Autodesk Inventor part; units mm, degrees
ref_plane "to_rail_XY" through (0.6, 10, 200) normal (0, 0, 1) x (1, 0, 0)
ref_plane "to_rail_YZ" through (0.6, 10, 200) normal (1, 0, 0) x (0, 1, 0)
ref_plane "to_rail_ZX" through (0.6, 10, 200) normal (0, 1, 0) x (0, 0, 1)
sketch "Sketch_1" plane through (0, 0, 0) normal (0, 0, 1) x (1, 0, 0)
  line L0 (-7.4, 19.7) -> (-7.4, 0.3)
  arc A0 (-7.4, 0.3) -> (-7.1, 0) centre (-7.1, 0.3) ccw
  line L1 (-7.1, 0) -> (-0.3, 0)
  arc A1 (-0.3, 0) -> (0, 0.3) centre (-0.3, 0.3) ccw
  line L2 (0, 0.3) -> (0, 2.95)
  arc A2 (0, 2.95) -> (-0.2, 3.15) centre (-0.2, 2.95) ccw
  line L3 (-0.2, 3.15) -> (-0.5141, 3.15)
  arc A3 (-0.5141, 3.15) -> (-0.708, 2.999) centre (-0.5141, 2.95) ccw
  arc A4 (-4.392, 2.999) -> (-0.708, 2.999) centre (-2.55, 3.465) ccw
  arc A5 (-4.392, 2.999) -> (-4.5859, 3.15) centre (-4.5859, 2.95) ccw
  line L4 (-4.5859, 3.15) -> (-5.8, 3.15)
  arc A6 (-6, 3.35) -> (-5.8, 3.15) centre (-5.8, 3.35) ccw
  line L5 (-6, 3.35) -> (-6, 16.65)
  arc A7 (-5.8, 16.85) -> (-6, 16.65) centre (-5.8, 16.65) ccw
  line L6 (-5.8, 16.85) -> (-4.5859, 16.85)
  arc A8 (-4.5859, 16.85) -> (-4.392, 17.001) centre (-4.5859, 17.05) ccw
  arc A9 (-0.708, 17.001) -> (-4.392, 17.001) centre (-2.55, 16.535) ccw
  arc A10 (-0.708, 17.001) -> (-0.5141, 16.85) centre (-0.5141, 17.05) ccw
  line L7 (-0.5141, 16.85) -> (-0.2, 16.85)
  arc A11 (-0.2, 16.85) -> (0, 17.05) centre (-0.2, 17.05) ccw
  line L8 (0, 17.05) -> (0, 19.7)
  arc A12 (0, 19.7) -> (-0.3, 20) centre (-0.3, 19.7) ccw
  line L9 (-0.3, 20) -> (-7.1, 20)
  arc A13 (-7.1, 20) -> (-7.4, 19.7) centre (-7.1, 19.7) ccw
extrude "Extrusion1" add sketch "Sketch_1" along normal blind 400
sketch "Sketch2" plane through (-6, 3.35, 0) normal (1, 0, 0) x (0, 0, -1)
  point P0 (-15, 6.65)
hole "Hole1" at (-6, 10, 15) direction (-1, 0, 0) diameter 3.5 depth 1.4 countersink diameter 6.1 countersink angle 90
pattern_linear "Rectangular Pattern1" count 3 spacing 185 along (0, 0, 1) of "Hole1"
ref_plane "to_rail_XY" through (0.6, 10, 200) normal (0, 0, 1) x (1, 0, 0)
ref_plane "to_rail_YZ" through (0.6, 10, 200) normal (1, 0, 0) x (0, 1, 0)
ref_plane "to_rail_ZX" through (0.6, 10, 200) normal (0, 1, 0) x (0, 0, 1)
properties part number "SAR340-40_b"
Check sheet for the modelled part. Datum: model origin and axes. Units: mm. Coordinates: 2 decimals unless noted, no trailing zeros. Write each loop counter-clockwise with the first axis right and the second up, starting at its lowest first coordinate (ties: lowest second). Pieces come first, ordered by that corner, then holes. Notation, with made-up numbers: M -6.75,73 L 3.25,73 A32 cw 3.25,101 Z; hole C 12.25,63 d3. An arc over 180 degrees is marked long. Write item = value, one per line. Start each with the question number.
1. Go/stop test with flat-tipped pins: pin 1 (3 mm diameter, centred on y = 10, z = 200, fed in from +X); pin 2 (4 mm diameter, centred on y = 10, z = 211, fed in from +X). Record where each tip stops, or that it passes through.
2. Sectioned sample at B-B (z = 137.5). Record the cut outline in (x, y) (3 decimals).
3. Sectioned sample at A-A (x = -2.5). Record the cut outline in (y, z), then the cut area to 3 significant figures.
4. Thickness scan on probe 1 along Z at (x, y) = (-7.25, 10); probe 2 along Z at (x, y) = (-7.35, 10); probe 3 along Y at (x, z) = (-7.3, 385). Record the ranges inside material, lowest first.
5. Mould release check, pull along Y, two halves, no side actions. Record for faces 1 (the flat face through (-6, 8, 197)), 2 (the flat face through (-7.4, 10, 197)), 3 (the flat face through (-4, 20, 197)): pulls with the +Y half, pulls with the -Y half, needs draft (parallel to the pull), parting line crosses it, or undercut.
The answers:
q1.pin_1 = through
q1.pin_2 = -6
q2.outline = M -7.4,0.3 A0.3 ccw -7.1,0 L -0.3,0 A0.3 ccw 0,0.3 L 0,2.95 A0.2 ccw -0.2,3.15 L -0.514,3.15 A0.2 ccw -0.708,2.999 A1.9 cw -4.392,2.999 A0.2 ccw -4.586,3.15 L -5.8,3.15 A0.2 cw -6,3.35 L -6,16.65 A0.2 cw -5.8,16.85 L -4.586,16.85 A0.2 ccw -4.392,17.001 A1.9 cw -0.708,17.001 A0.2 ccw -0.514,16.85 L -0.2,16.85 A0.2 ccw 0,17.05 L 0,19.7 A0.3 ccw -0.3,20 L -7.1,20 A0.3 ccw -7.4,19.7 Z
q3.outline = M 0,0 L 1.57,0 L 1.57,400 L 0,400 Z; M 18.43,0 L 20,0 L 20,400 L 18.43,400 Z
q3.area = 1,250 mm²
q4.probe_1 = 0 to 13.2, 16.8 to 198.2, 201.8 to 383.2, 386.8 to 400
q4.probe_2 = 0 to 13.25, 16.75 to 198.25, 201.75 to 383.25, 386.75 to 400
q4.probe_3 = 0.08 to 8.25, 11.75 to 19.92
q5.face_1 = undercut
q5.face_2 = needs draft
q5.face_3 = pulls with the +Y half
